Part model, mm, in its own coordinate system. Round coordinates to 2 decimals unless told otherwise and drop trailing zeros. Write each loop counter-clockwise with the first axis right and the second up, starting at its lowest first coordinate (ties: lowest second). Pieces come first, ordered by that corner, then holes. Notation, with made-up numbers: (48.25, 16.25) -> (99.25, 16.25) arc R14 ccw to (99.25, 27.25) -> close; hole circle Ø6 at (15.5, 46.25). An arc over 180 degrees is marked (long way). Return JSON: item names as keys, results as strings. Group by question number.
(1) Saw through at A-A (y = 2.1). State how many separate pieces and enclosed holes the cut face has, plus the area to 3 significant figures.
(2) Saw through at B-B (z = -2). List the corners of the cut face in (x, y).
(3) Saw through at C-C (z = -15.75). List the corners of the cut face in (x, y).
(4) Drill centre lines: L1, parallel to X at y = 2, z = -10; L2, parallel to X at y = 2, z = -7.5; L3, parallel to Z at x = 11, y = 3. Where is each one in solid material? Low to high. Write a range as from..to.
(5) Drop a flat-ended pin along its axis: pin 1 Ø2 at (y, z) = (5, -17) entering from -X. Give the stop position or say it passes through.
from build123d import *

# Parameters (mm, degrees)
SKETCH2_W           = 200
SKETCH2_H           = 20
BOSS_EXTRUDE1_DEPTH = 6
SKETCH3_R           = 3
CUT_EXTRUDE1_DEPTH  = 202.087045828
SKETCH4_R           = 3
CUT_EXTRUDE2_DEPTH  = 202.087045828
FILLET1_R           = 10
FILLET2_R           = 10
SKETCH6_R           = 3
CUT_EXTRUDE3_DEPTH  = 202.087045828


with BuildPart() as part:
    # Sketch2 → Boss-Extrude1 (new body)
    with BuildSketch(Plane(origin=(0, 0, 0), x_dir=(1, 0, 0), z_dir=(0, 1, 0))):
        with Locations((100, 10)):
            Rectangle(SKETCH2_W, SKETCH2_H)
    extrude(amount=BOSS_EXTRUDE1_DEPTH)

    # Sketch3 → Cut-Extrude1 (cut, through all)
    with BuildSketch(Plane(origin=(0, 6, 0), x_dir=(1, 0, 0), z_dir=(0, 1, 0))):
        with Locations(Location((9, 10, 0), (0, 0, 270))):
            Circle(SKETCH3_R)
    extrude(amount=-CUT_EXTRUDE1_DEPTH, mode=Mode.SUBTRACT)

    # Sketch4 → Cut-Extrude2 (cut, through all)
    with BuildSketch(Plane(origin=(0, 6, 0), x_dir=(1, 0, 0), z_dir=(0, 1, 0))):
        with Locations(Location((191, 10, 0), (0, 0, 270))):
            Circle(SKETCH4_R)
    extrude(amount=-CUT_EXTRUDE2_DEPTH, mode=Mode.SUBTRACT)

    # Fillet1
    fillet1_edges = [part.edges().sort_by_distance(p)[0] for p in [
        (0, 3, -20),
        (0, 3, 0),
    ]]
    fillet(fillet1_edges, radius=FILLET1_R - 0.0001)  # a hair under: the kernel refuses the full size

    # Fillet2
    fillet2_edges = [part.edges().sort_by_distance(p)[0] for p in [
        (200, 3, -20),
        (200, 3, 0),
    ]]
    fillet(fillet2_edges, radius=FILLET2_R - 0.0001)  # a hair under: the kernel refuses the full size

    # Sketch6 → Cut-Extrude3 (cut, through all)
    with BuildSketch(Plane(origin=(0, 6, 0), x_dir=(1, 0, 0), z_dir=(0, 1, 0))):
        with Locations(Location((100, 10, 0), (0, 0, 270))):
            Circle(SKETCH6_R)
    extrude(amount=-CUT_EXTRUDE3_DEPTH, mode=Mode.SUBTRACT)


solid = part.part
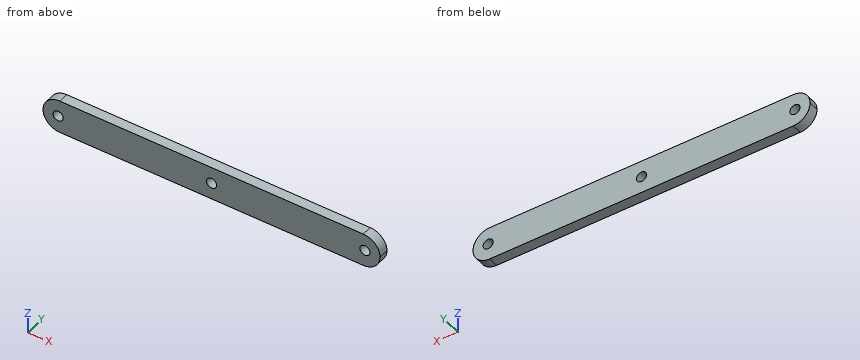
Computed values:
{
 "1": {"separate pieces": "1", "enclosed holes": "3", "area": "3,830 mm2"},
 "2": {"outline": "(4, 0) -> (196, 0) -> (196, 6) -> (4, 6) -> close"},
 "3": {"outline": "(1.82, 0) -> (198.18, 0) -> (198.18, 6) -> (1.82, 6) -> close"},
 "4": {"L1": "0..6, 12..97, 103..188, 194..200", "L2": "0.32..7.34, 10.66..98.34, 101.66..189.34, 192.66..199.68", "L3": "-20..-12.24, -7.76..0"},
 "5": {"pin 1": "x = 2"}
}
